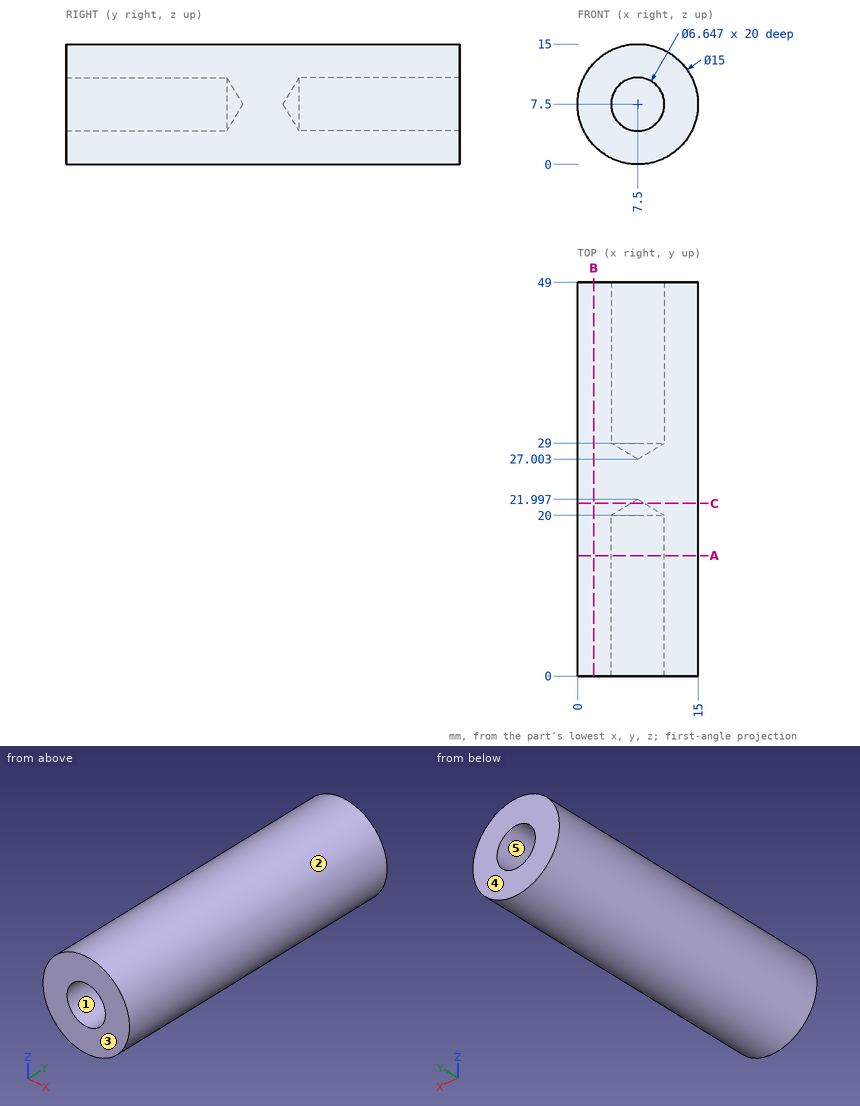
The drawing under review shows one solid part. Ordinate dimensions are in mm from its lowest x, y, z. A direction names the side the tool comes from. Round coordinates to 2 decimals unless told otherwise and drop trailing zeros. Loops run counter-clockwise (first coordinate to the right, second up) from the corner with the lowest first, then second, coordinate; pieces in that order, holes last. Notation, with made-up numbers: (-12.5, 27.5) - (10.5, 27.5) arc R12 ccw to (10.5, 37.5) - close; hole circle Ø5 at (-9, -5.75). An arc over 180 degrees is marked (long way). Use one line per item in the form item = value.
Item 1: Mouldability with a two-part tool opening along Z and no side actions: class the marked faces 1, 2 and 3 as +Z half, -Z half, draft (parallel to the pull), parting line (faces both ways), or undercut.
Answers:
face_1 = undercut
face_2 = parting line
face_3 = draft
Item 2: For line 1 (Z direction, x = 7.5, y = 15); line 2 (X direction, y = 39, z = 8.5); line 3 (X direction, y = 11, z = 4.75), list the stretches that pass through material, from the lowest coordinate up.
Answers:
line_1 = 0 to 4.18, 10.82 to 15
line_2 = 0.07 to 4.33, 10.67 to 14.93
line_3 = 0.52 to 5.63, 9.37 to 14.48
Item 3: Consider section C-C on y = 21.5. Write out the cut boundary in (x, z), then the cut area to 3 significant figures.
Answers:
outline = circle Ø15 at (7.5, 7.5); hole circle Ø1.65 at (7.5, 7.5)
area = 175 mm^2
Item 4: Consider section B-B on x = 2. Write out the cut boundary in (y, z), then the cut area to 3 significant figures.
Answers:
outline = (0, 2.4) - (49, 2.4) - (49, 12.6) - (0, 12.6) - close
area = 500 mm^2
Item 5: Clearance check with flat-ended pins moving along their axes: P1, Ø1.5, axis at y = 34, z = 5.5, coming from the +X side; P2, Ø5.5, axis at x = 7.5, z = 7.5, coming from the +Y side; P3, Ø4, axis at x = 7.5, z = 7.5, coming from the -Y side. State where each tip first meets the part, or that it passes through.
Answers:
P1 = 14.9
P2 = 28.66
P3 = 20.8
Item 6: Tool access review of the marked faces 4 and 5: name each direction out of +Z, -Z, +X, -X, +Y, -Y from which nothing blocks a thin tool from reaching the whole face with its end or side.
Answers:
face_4 = +Z, -Z, +X, -X, +Y
face_5 = +Y
Item 7: Consider section A-A on y = 15. Write out the cut boundary in (x, z), then the cut area to 3 significant figures.
Answers:
outline = circle Ø15 at (7.5, 7.5); hole circle Ø6.65 at (7.5, 7.5)
area = 142 mm^2
